Source: CAD feature listing. Evaluate the final solid. Frame: model axes, mm. Face numbers are marked on the shaded views. A direction names the side the tool comes from. Coordinates: 2 decimals unless noted, no trailing zeros. Order: outer loops, then holes, each group sorted by start corner. A loop starts at its lowest first (then second) coordinate and runs counter-clockwise, first axis right, second up.
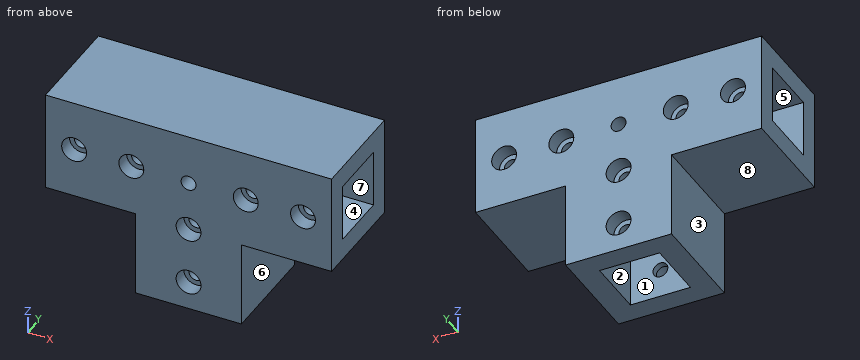
```python
from build123d import *

# Parameters (mm, degrees)
F0_W      = 100
F0_H      = 36
F1_DEPTH  = 7.5
F2_W      = 100
F2_H      = 7.5
F3_DEPTH  = 20
F4_W      = 100
F4_H      = 36
F4_W_2    = 21
F4_H_2    = 21
F5_DEPTH  = 7.5
F6_W      = 37
F6_H      = 36
F6_W_2    = 21
F6_H_2    = 21
F7_DEPTH  = 30
F8_R      = 2.6
F9_DEPTH  = 60
F10_R     = 4.35
F11_DEPTH = 5.25
F12_R     = 4.35
F13_DEPTH = 5.25


with BuildPart() as f1:
    # F0 (on Top) → F1 (new body)
    with BuildSketch(Plane.XY):
        with Locations((-50, 18)):
            Rectangle(F0_W, F0_H)
    extrude(amount=F1_DEPTH)

    # F2 (on face) → F3 (join)
    with BuildSketch(Plane(origin=(0, 0, 0), x_dir=(1, 0, 0), z_dir=(0, 0, -1))):
        with Locations((-50, -3.75)):
            Rectangle(F2_W, F2_H)
        with Locations((-50, -32.25)):
            Rectangle(F2_W, F2_H)
    extrude(amount=F3_DEPTH)

    # F4 (on face) → F5 (join)
    with BuildSketch(Plane(origin=(0, 0, -20), x_dir=(1, 0, 0), z_dir=(0, 0, -1))):
        with Locations((-50, -18)):
            Rectangle(F4_W, F4_H)
        with Locations((-50, -18)):
            Rectangle(F4_W_2, F4_H_2, mode=Mode.SUBTRACT)
    extrude(amount=F5_DEPTH)

    # F6 (on face) → F7 (join)
    with BuildSketch(Plane(origin=(0, 0, -27.5), x_dir=(1, 0, 0), z_dir=(0, 0, -1))):
        with Locations((-50, -18)):
            Rectangle(F6_W, F6_H)
        with Locations((-50, -18)):
            Rectangle(F6_W_2, F6_H_2, mode=Mode.SUBTRACT)
    extrude(amount=F7_DEPTH)

    # F8 (on face) → F9 (cut)
    with BuildSketch(Plane.XZ):
        with Locations((-90, -10)):
            Circle(F8_R)
        with Locations((-50, -10)):
            Circle(F8_R)
        with Locations((-10, -10)):
            Circle(F8_R)
        with Locations((-30, -10)):
            Circle(F8_R)
        with Locations((-70, -10)):
            Circle(F8_R)
        with Locations((-50, -47.5)):
            Circle(F8_R)
        with Locations((-50, -27.5)):
            Circle(F8_R)
    extrude(amount=-F9_DEPTH, mode=Mode.SUBTRACT)

    # F10 (on face) → F11 (cut)
    with BuildSketch(Plane(origin=(0, 36, 0), x_dir=(-1, 0, 0), z_dir=(0, 1, 0))):
        with Locations((50, -47.5)):
            Circle(F10_R)
        with Locations((50, -27.5)):
            Circle(F10_R)
        with Locations((90, -10)):
            Circle(F10_R)
        with Locations((70, -10)):
            Circle(F10_R)
        with Locations((30, -10)):
            Circle(F10_R)
        with Locations((10, -10)):
            Circle(F10_R)
    extrude(amount=-F11_DEPTH, mode=Mode.SUBTRACT)

    # F12 (on face) → F13 (cut)
    with BuildSketch(Plane.XZ):
        with Locations((-90, -10)):
            Circle(F12_R)
        with Locations((-70, -10)):
            Circle(F12_R)
        with Locations((-30, -10)):
            Circle(F12_R)
        with Locations((-10, -10)):
            Circle(F12_R)
        with Locations((-50, -27.5)):
            Circle(F12_R)
        with Locations((-50, -47.5)):
            Circle(F12_R)
    extrude(amount=-F13_DEPTH, mode=Mode.SUBTRACT)


solid = f1.part
```
Q1. Pin query (flat end, axial travel): P1, Ø1, axis at y = 21.5, z = -30, coming from the -X side; P2, Ø4.5, axis at x = -48, z = -47, coming from the -Y side; P3, Ø12, axis at y = 7, z = -36, coming from the +X side. Return the tip coordinate at first contact, or that it passes through.
Solutions:
P1: stops at x = -68.5
P2: stops at y = 5.25
P3: stops at x = -31.5
Q2. Set-up query: the marked faces 5, 6, 7 and 8. Return all of +Z, -Z, +X, -X, +Y, -Y with unobstructed straight access to the full face (end or side cutting, diameter ignored); none if empty.
Solutions:
face 5: +X, -X
face 6: -Z, +X, +Y, -Y
face 7: none
face 8: -Z, -X, +Y, -Y
Q3. Section query D-D on x = -70. Output: boundary loops of the cut face in (y, z), plus the area to 3 significant figures.
Solutions:
outline: (0, -27.5) - (36, -27.5) - (36, -14.35) - (30.75, -14.35) - (30.75, -12.6) - (28.5, -12.6) - (28.5, -20) - (7.5, -20) - (7.5, -12.6) - (5.25, -12.6) - (5.25, -14.35) - (0, -14.35) - close; (0, -5.65) - (5.25, -5.65) - (5.25, -7.4) - (7.5, -7.4) - (7.5, 0) - (28.5, 0) - (28.5, -7.4) - (30.75, -7.4) - (30.75, -5.65) - (36, -5.65) - (36, 7.5) - (0, 7.5) - close
area: 725 mm2
Q4. Material intervals for line 1 along Z through (x, y) = (-50, 5.8); line 2 along Y through (x, z) = (-22.5, -12); line 3 along X through (y, z) = (24, -49), sorted ascending.
Solutions:
line 1: z = -57.5 to -50.1, -44.9 to -30.1, -24.9 to -12.6, -7.4 to 7.5
line 2: y = 0 to 7.5, 28.5 to 36
line 3: x = -68.5 to -60.5, -39.5 to -31.5
Q5. Section query B-B on x = -18. Output: boundary loops of the cut face in (y, z).
Solutions:
outline: (0, -27.5) - (36, -27.5) - (36, 7.5) - (0, 7.5) - close; hole (7.5, -20) - (28.5, -20) - (28.5, 0) - (7.5, 0) - close
Q6. Section query C-C on z = -38.5. Output: boundary loops of the cut face in (x, y).
Solutions:
outline: (-68.5, 0) - (-31.5, 0) - (-31.5, 36) - (-68.5, 36) - close; hole (-60.5, 7.5) - (-39.5, 7.5) - (-39.5, 28.5) - (-60.5, 28.5) - close
Q7. Pull-direction query (X, two-part tool) for the marked faces 1, 2, 3 and 4; classes: pulls with the +X half, pulls with the -X half, needs draft (parallel to the pull), parting line crosses it, or undercut.
Solutions:
face 1: undercut
face 2: undercut
face 3: pulls with the -X half
face 4: needs draft
Q8. Section query A-A on y = 3.5. Output: boundary loops of the cut face in (x, z).
Solutions:
outline: (-100, -27.5) - (-68.5, -27.5) - (-68.5, -57.5) - (-31.5, -57.5) - (-31.5, -27.5) - (0, -27.5) - (0, 7.5) - (-100, 7.5) - close; hole circle Ø8.7 at (-90, -10); hole circle Ø8.7 at (-70, -10); hole circle Ø8.7 at (-50, -47.5); hole circle Ø8.7 at (-50, -27.5); hole circle Ø5.2 at (-50, -10); hole circle Ø8.7 at (-30, -10); hole circle Ø8.7 at (-10, -10)
